Source: CAD feature listing. Evaluate the final solid. Frame: model axes, mm. A direction names the side the tool comes from. Give positions to 0.01 mm unless a question says otherwise; leave off trailing zeros. Write each loop counter-clockwise with the first axis right and the second up, starting at its lowest first coordinate (ties: lowest second). Pieces come first, ordered by that corner, then holes. Notation, with made-up numbers: (-10, -12) -> (26, -12) arc R20 cw to (26, -6) -> close; hole circle Ø6 at (-1, -28.5). An arc over 180 degrees is marked (long way). Write item = value, one per line.
from build123d import *

# Parameters (mm, degrees)
SKETCH1_W           = 150
SKETCH1_H           = 150
BOSS_EXTRUDE1_DEPTH = 55
SKETCH2_W           = 148
SKETCH2_H           = 148
CUT_EXTRUDE1_DEPTH  = 54
SKETCH3_W           = 132
SKETCH3_H           = 132
CUT_EXTRUDE2_DEPTH  = 2
SKETCH6_R           = 2.5
BOSS_EXTRUDE5_DEPTH = 5
SKETCH9_R           = 1.4
CUT_EXTRUDE4_DEPTH  = 10
CIRPATTERN1_COUNT   = 4


with BuildPart() as part:
    # Sketch1 → Boss-Extrude1 (new body)
    with BuildSketch(Plane(origin=(0, 0, 0), x_dir=(1, 0, 0), z_dir=(0, 1, 0))):
        Rectangle(SKETCH1_W, SKETCH1_H)
    extrude(amount=-BOSS_EXTRUDE1_DEPTH)

    # Sketch2 → Cut-Extrude1 (cut)
    with BuildSketch(Plane(origin=(0, 0, 0), x_dir=(1, 0, 0), z_dir=(0, 1, 0))):
        Rectangle(SKETCH2_W, SKETCH2_H)
    extrude(amount=-CUT_EXTRUDE1_DEPTH, mode=Mode.SUBTRACT)

    # Sketch3 → Cut-Extrude2 (cut, through all)
    with BuildSketch(Plane(origin=(0, -54, 0), x_dir=(1, 0, 0), z_dir=(0, 1, 0))):
        Rectangle(SKETCH3_W, SKETCH3_H)
    extrude(amount=-CUT_EXTRUDE2_DEPTH, mode=Mode.SUBTRACT)

    # Sketch6 → Boss-Extrude5 (add)
    with BuildSketch(Plane.XZ.offset(55)):
        with Locations((-70.678187872, -25)):
            Circle(SKETCH6_R)
        with Locations((-70.678187872, 25)):
            Circle(SKETCH6_R)
        with Locations((25, 70.678187872)):
            Circle(SKETCH6_R)
        with Locations((-25, 70.678187872)):
            Circle(SKETCH6_R)
        with Locations((70.678187872, -25)):
            Circle(SKETCH6_R)
        with Locations((70.678187872, 25)):
            Circle(SKETCH6_R)
        with Locations((-25, -70.678187872)):
            Circle(SKETCH6_R)
        with Locations((25, -70.678187872)):
            Circle(SKETCH6_R)
    extrude(amount=BOSS_EXTRUDE5_DEPTH)

    # Sketch9 → Cut-Extrude4 (cut)
    with BuildSketch(Plane.ZY.offset(75)):
        with Locations((-6.1, -7.25)):
            Circle(SKETCH9_R)
        with Locations((6.1, -7.25)):
            Circle(SKETCH9_R)
        with Locations((6.1, -15.25)):
            Circle(SKETCH9_R)
        with Locations((-6.1, -15.25)):
            Circle(SKETCH9_R)
    cut_extrude4 = extrude(amount=-CUT_EXTRUDE4_DEPTH, mode=Mode.SUBTRACT)

    # CirPattern1: Cut-Extrude4 ×4 about axis
    cirpattern1_axis = Axis((0, 0, 0), (0, 1, 0))
    for i in range(1, CIRPATTERN1_COUNT):
        add(cut_extrude4.rotate(cirpattern1_axis, i * 360 / CIRPATTERN1_COUNT), mode=Mode.SUBTRACT)


solid = part.part
1) Cut plane C-C (y = -33.5). Return the cut outline in (x, z), then the cut area to 3 significant figures.
Computed:
outline = (-75, -75) -> (75, -75) -> (75, 75) -> (-75, 75) -> close; hole (-74, -74) -> (74, -74) -> (74, 74) -> (-74, 74) -> close
area = 596 mm²
2) Draft query along X for faces 4 (the flat face through (-1, -27, -74)), 5 (the flat face through (75, -27, 1)), 6 (the flat face through (-75, -27, 1)), 7 (the flat face through (-1, -27, 75)). Return one class per face: pulls with the +X half, pulls with the -X half, needs draft (parallel to the pull), parting line crosses it, or undercut.
Computed:
face_4 = undercut
face_5 = pulls with the +X half
face_6 = pulls with the -X half
face_7 = needs draft
3) Cut plane B-B (x = -58.5). Return the cut outline in (y, z), then the cut area to 3 significant figures.
Computed:
outline = (-55, -75) -> (0, -75) -> (0, -74) -> (-54, -74) -> (-54, -66) -> (-55, -66) -> close; (-55, 66) -> (-54, 66) -> (-54, 74) -> (0, 74) -> (0, 75) -> (-55, 75) -> close
area = 126 mm²
4) Cut plane A-A (z = -25). Return the cut outline in (x, y).
Computed:
outline = (-75, -55) -> (-73.18, -55) -> (-73.18, -60) -> (-68.18, -60) -> (-68.18, -55) -> (-66, -55) -> (-66, -54) -> (-74, -54) -> (-74, 0) -> (-75, 0) -> close; (66, -55) -> (68.18, -55) -> (68.18, -60) -> (73.18, -60) -> (73.18, -55) -> (75, -55) -> (75, 0) -> (74, 0) -> (74, -54) -> (66, -54) -> close
5) Material intervals for L1, parallel to Y at x = -74.5, z = -6.1; L2, parallel to X at y = -42.5, z = 44, sorted ascending.
Computed:
L1 = -55 to -16.65, -13.85 to -8.65, -5.85 to 0
L2 = -75 to -74, 74 to 75
6) Cut plane D-D (z = 46.5). Return the cut outline in (x, y), then the cut area to 3 significant figures.
Computed:
outline = (-75, -55) -> (-66, -55) -> (-66, -54) -> (-74, -54) -> (-74, 0) -> (-75, 0) -> close; (66, -55) -> (75, -55) -> (75, 0) -> (74, 0) -> (74, -54) -> (66, -54) -> close
area = 126 mm²
7) Access query for faces 1 (the flat face through (-71, -60, 25)), 2 (the flat face through (-1, -27, 74)), 3 (the cylindrical face through (73.063, -57.465, 25.751)). Directions: +Z, -Z, +X, -X, +Y, -Y. A direction counts if a zero-diameter tool reaches every point of the face in a straight line with its end or side. Return the directions, or none.
Computed:
face_1 = +Z, -Z, +X, -X, -Y
face_2 = +Y
face_3 = -Y
